Verification items for the finished model (mm, model axes). A direction names the side the tool comes from. Round coordinates to 2 decimals unless told otherwise and drop trailing zeros. Order: outer loops, then holes, each group sorted by start corner. A loop starts at its lowest first (then second) coordinate and runs counter-clockwise, first axis right, second up. Notation, with made-up numbers: M 82,89.5 L 120,89.5 A16 cw 120,102.5 Z; hole C -2.5,30 d1. An arc over 180 degrees is marked long. Use one line per item in the form item = value. Start each with the question number.
Item 1: Release check for a two-part mould opening along Y. For faces 4 (the flat face through (-13, 60, 69)), 5 (the cylindrical face through (-2.46, 33.08, 71.25)), 6 (the flat face through (-7, 44, 80)) record: +Y half, -Y half, draft (parallel to the pull), parting line (faces both ways), or undercut.
Item 2: Thickness scan on probe 1 along Z at (x, y) = (-13.25, 50); probe 2 along Y at (x, z) = (-1.5, 75); probe 3 along Z at (x, y) = (-10.75, 46). Record the ranges inside material, lowest first. Write a range as [from, to].
Item 3: Cross-section at A-A on x = -3.75. Enter the section's corners in (y, z), then the cut area to 3 significant figures.
Item 4: Cross-section at B-B on y = 52. Enter the section's corners in (x, z), then the cut area to 3 significant figures.
Item 5: Tool access check on faces 1 (the cylindrical face through (-11.49, 41.54, 68.5)), 2 (the flat face through (-5, 40, 7)), 3 (the flat face through (-13, 55, 22.5)). Record the directions out of +Z, -Z, +X, -X, +Y, -Y that give a thin tool (end or side, any length) a straight path to the whole face; none if there is none.
Item 6: Cross-section at C-C on z = 38. Enter the section's corners in (x, y).
Item 7: Go/stop test with flat-tipped pins: pin 1 Ø8 at (x, z) = (-7.5, 54.5) entering from -Y; pin 2 Ø12 at (y, z) = (39.43, 10.16) entering from -X; pin 3 Ø4 at (y, z) = (40.5, 73) entering from +X. Record where each tip stops, or that it passes through.
Item 8: Cross-section at D-D on z = 20.5. Enter the section's corners in (x, y).
from build123d import *

# Parameters (mm, degrees)
BOSS_EXTRU_1_DEPTH      = 80
ENL_V_MAT_EXTRU_1_DEPTH = 104.324730825
ESQUISSE4_R             = 2.5
ENL_V_MAT_EXTRU_2_DEPTH = 80
ESQUISSE6_R             = 6.505119939
ESQUISSE6_R_2           = 6.755806102
ENL_V_MAT_EXTRU_3_DEPTH = 5


with BuildPart() as part:
    # Esquisse2 → Boss.-Extru.1 (new body)
    with BuildSketch(Plane.XY):
        Polygon((0, 0), (0, 60), (-26, 60), align=None)
    extrude(amount=BOSS_EXTRU_1_DEPTH)

    # Esquisse3 → Enlèv. mat.-Extru.1 (cut, through all)
    with BuildSketch(Plane(origin=(0, 0, 0), x_dir=(0, 0, -1), z_dir=(1, 0, 0))):
        with BuildLine():
            Line((-57.5, 50), (-57.5, 60))
            Line((-57.5, 60), (-22.5, 60))
            Line((-22.5, 60), (-22.5, 50))
            ThreePointArc((-22.5, 50), (-40, 32.5), (-57.5, 50))
        make_face()
    extrude(amount=-ENL_V_MAT_EXTRU_1_DEPTH, mode=Mode.SUBTRACT)

    # Esquisse4 → Enlèv. mat.-Extru.2 (cut)
    with BuildSketch(Plane(origin=(0, 0, 0), x_dir=(0, 0, -1), z_dir=(1, 0, 0))):
        with Locations((-69.841791115, 39.429492972)):
            Circle(ESQUISSE4_R)
        with Locations((-10.158208885, 39.429492972)):
            Circle(ESQUISSE4_R)
    extrude(amount=-ENL_V_MAT_EXTRU_2_DEPTH, mode=Mode.SUBTRACT)

    # Esquisse6 → Enlèv. mat.-Extru.3 (cut)
    with BuildSketch(Plane(origin=(0, 0, 0), x_dir=(0, 0, -1), z_dir=(1, 0, 0))):
        with Locations((-69.841791115, 39.429492972)):
            Circle(ESQUISSE6_R)
        with Locations((-10.158208885, 39.429492972)):
            Circle(ESQUISSE6_R_2)
    extrude(amount=-ENL_V_MAT_EXTRU_3_DEPTH, mode=Mode.SUBTRACT)


solid = part.part
Output values:
q1.face_4 = +Y half
q1.face_5 = undercut
q1.face_6 = draft
q2.probe_1 = [0, 22.5], [57.5, 80]
q2.probe_2 = [3.46, 35.47], [43.39, 60]
q2.probe_3 = [0, 22.96], [57.04, 80]
q3.outline = M 8.65,0 L 60,0 L 60,22.5 L 50,22.5 A17.5 cw 50,57.5 L 60,57.5 L 60,80 L 8.65,80 Z; hole C 39.43,10.16 d13.51; hole C 39.43,69.84 d13.01
q3.area = 3,000 mm2
q4.outline = M -22.53,0 L 0,0 L 0,22.5 L -22.53,22.5 Z; M -22.53,57.5 L 0,57.5 L 0,80 L -22.53,80 Z
q4.area = 1,010 mm2
q5.face_1 = +X, -X
q5.face_2 = +X
q5.face_3 = +X, -X, +Y
q6.outline = M -14.13,32.61 L 0,0 L 0,32.61 Z
q7.pin_1 = 8.08
q7.pin_2 = -19.69
q7.pin_3 = -5
q8.outline = M -26,60 L 0,0 L 0,60 Z
